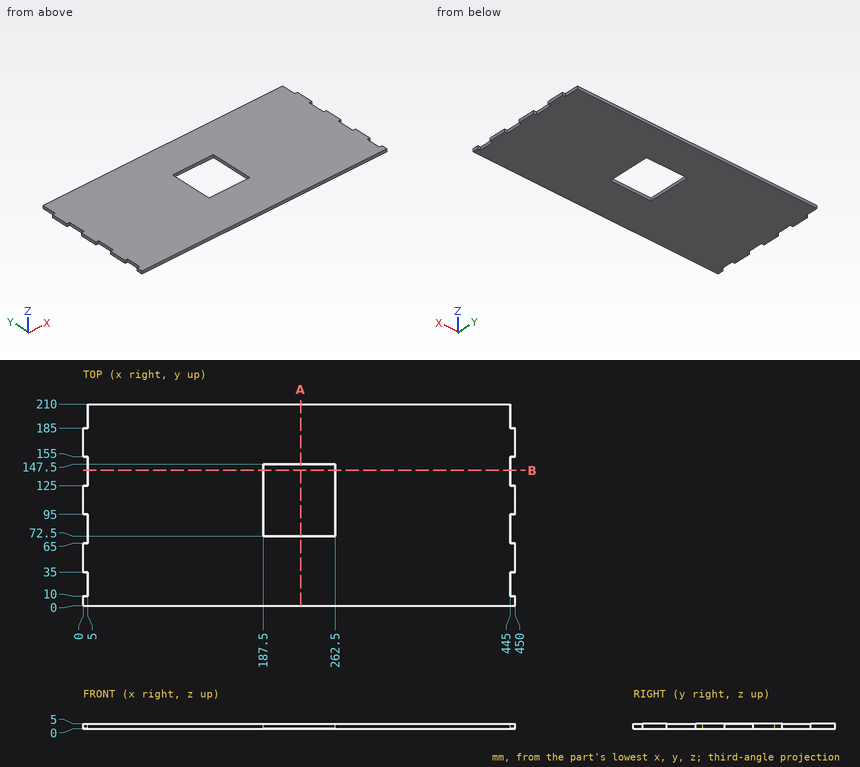
Design review of the part shown in the three views and the two pictorial views. Dimensions are in mm from the part's minimum x, y and z. Round coordinates to 2 decimals unless told otherwise and drop trailing zeros. Loops run counter-clockwise (first coordinate to the right, second up) from the corner with the lowest first, then second, coordinate; pieces in that order, holes last.
1) Consider section B-B on y = 141. State the section outline as (x, z) points.
Values follow:
outline: (5, 0) - (187.5, 0) - (187.5, 5) - (5, 5) - close; (262.5, 0) - (445, 0) - (445, 5) - (262.5, 5) - close
2) Clearance check with flat-ended pins moving along their axes: P1, Ø1.5, axis at x = 3, z = 2, coming from the +Y side; P2, Ø1.5, axis at y = 145, z = 3, coming from the +X side. State where each tip first meets the part, or that it passes through.
Values follow:
P1: stops at y = 185
P2: stops at x = 445
3) Wall thickness on line 1 along X through (y, z) = (131.5, 3.5); line 2 along X through (y, z) = (108.5, 2.25); line 3 along X through (y, z) = (28, 2.9): over which ranges is each line inside the solid? List them lowest first.
Values follow:
line 1: x = 5 to 187.5, 262.5 to 445
line 2: x = 0 to 187.5, 262.5 to 450
line 3: x = 5 to 445
4) Consider section A-A on x = 226.5. State the section outline as (y, z) points, then the cut area to 3 significant figures.
Values follow:
outline: (0, 0) - (72.5, 0) - (72.5, 5) - (0, 5) - close; (147.5, 0) - (210, 0) - (210, 5) - (147.5, 5) - close
area: 675 mm2
